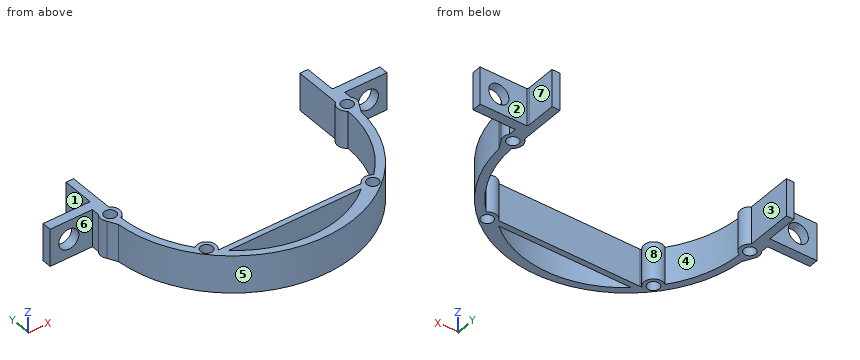
Autodesk Inventor part; units mm, degrees
ref_plane "YZ Plane" through (0, 0, 0) normal (1, 0, 0) x (0, 1, 0)
ref_plane "XZ Plane" through (0, 0, 0) normal (0, 1, 0) x (-1, 0, 0)
ref_plane "XY Plane" through (0, 0, 0) normal (0, 0, 1) x (1, 0, 0)
sketch "Esquisse1" plane through (0, 0, 0) normal (0, 0, 1) x (1, 0, 0)
  line L0 (0, 0) -> (-27.546, -25.0426) construction
  line L1 (0, 0) -> (23.0277, -27.4577) construction
  circle A0 centre (-18.0975, -16.4528) radius 1.25
  circle A1 centre (15.7127, -18.7355) radius 1.25
  arc A2 (-16.6894, -17.8731) -> (14.1299, -19.9581) centre (0, 0) ccw
  arc A3 (-16.6894, -17.8731) -> (-19.3824, -14.9201) centre (-18.0975, -16.4528) ccw
  arc A4 (17.0433, -17.2424) -> (14.1299, -19.9581) centre (15.7127, -18.7355) ccw
  line L2 (0, 0) -> (-29.5508, 10.7556) construction
  line L3 (-17.8311, 0) -> (17.1748, 0) construction
  line L4 (0, 2.0526) -> (0, -2.2236) construction
  arc A5 (-25.923, -2) -> (25.923, -2) centre (0, 0) ccw
  circle A6 centre (0, 0) radius 22.5 construction
  arc A7 (-16.6894, -17.8731) -> (14.1299, -19.9581) centre (0, 0) ccw
  arc A8 (-16.6894, -17.8731) -> (14.1299, -19.9581) centre (0, 0) ccw
  circle A9 centre (-25.3169, 1.1605) radius 1.25
  circle A10 centre (25.3169, 1.1605) radius 1.25
  line L5 (24.0891, 2.7784) -> (24.0891, 12.8348)
  line L6 (25.8363, 12.8348) -> (24.0891, 12.8348)
  line L7 (-25.923, 6.143) -> (-25.923, 12.7847)
  line L8 (-24.2942, 2.9148) -> (-24.2942, 12.7847)
  line L9 (-24.2942, 12.7847) -> (-25.923, 12.7847)
  arc A11 (-24.4506, -0.676) -> (-19.3824, -14.9201) centre (0, 0) ccw
  arc A12 (-24.4506, -0.676) -> (-19.3824, -14.9201) centre (0, 0) ccw
  arc A13 (-24.4506, -0.676) -> (-24.2942, 2.9148) centre (-25.3169, 1.1605) ccw
  arc A14 (17.0433, -17.2424) -> (24.2376, -0.5599) centre (0, 0) ccw
  arc A15 (17.0433, -17.2424) -> (24.2376, -0.5599) centre (0, 0) ccw
  arc A16 (17.0433, -17.2424) -> (24.2376, -0.5599) centre (0, 0) ccw
  arc A17 (24.0891, 2.7784) -> (24.2376, -0.5599) centre (25.3169, 1.1605) ccw
  line L10 (25.8363, 3.0919) -> (25.8363, 3.124)
  line L11 (25.8363, 6.3239) -> (25.8363, 12.8348)
  line L12 (25.8363, 6.3239) -> (25.9915, 6)
  line L13 (-36, 4) -> (-26.9495, 4)
  line L14 (-36, 6) -> (-26, 6)
  line L15 (-36, 4) -> (-36, 6)
  line L16 (-26, 6) -> (-25.9915, 6)
  line L17 (-25.9915, 6) -> (-25.923, 6.143)
  line L18 (-26.9495, 4) -> (-26.9495, 2.3678)
  line L19 (-25.923, -2) -> (-26.9495, -0.0468)
  arc A18 (-26.9495, 2.3678) -> (-26.9495, -0.0468) centre (-25.3169, 1.1605) ccw
  arc A19 (-24.4506, -0.676) -> (-24.2942, 2.9148) centre (-25.3169, 1.1605) ccw
  line L20 (25.9915, 6) -> (25.923, 6.143)
  line L21 (36, 4) -> (26.9495, 4)
  line L22 (36, 6) -> (26, 6)
  line L23 (36, 4) -> (36, 6)
  line L24 (26.9495, 4) -> (26.9495, 2.3678)
  line L25 (25.923, -2) -> (26.9495, -0.0468)
  arc A20 (26.9495, -0.0468) -> (26.9495, 2.3678) centre (25.3169, 1.1605) ccw
  line L26 (25.9915, 6) -> (26, 6)
  point P0 (29.8237, -2)
  point P1 (-36, -2)
  point P2 (-26.3114, 9.5766)
  dimension "d35" = 2.5
  dimension "d36" = 2.5
  dimension "d37" = 4
  dimension "d38" = 4
  dimension "d39" = 20
  dimension "d52" = 45
  dimension "d65" = 2.5
  dimension "d81" = 10
ref_plane "Plan de construction1" through (-42, 0, 0) normal (0, 1, 0) x (1, 0, 0)
ref_plane "Plan de construction2" through (-36, 0, 0) normal (0, 1, 0) x (1, 0, 0)
sketch "Esquisse3" plane through (-36, 0, 0) normal (0, 1, 0) x (1, 0, 0)
  line L0 (0, 0) -> (10, 0)
  line L1 (0, 0) -> (0, -8)
  line L2 (10, -8) -> (0, -8)
  line L3 (10, 0) -> (10, -8)
  circle A0 centre (4, -4) radius 2.15
  line L4 (62, 0) -> (72, 0)
  line L5 (62, 0) -> (62, -8)
  line L6 (72, -8) -> (62, -8)
  line L7 (72, 0) -> (72, -8)
  circle A1 centre (68, -4) radius 2.15
  point P0 (36, 0)
  dimension "d48" = 4.3
  dimension "d73" = 4
  dimension "d74" = 4.3
  dimension "d75" = 4
extrude "Extrusion16" add sketch "Esquisse1" along normal blind 8
extrude "Extrusion17" cut sketch "Esquisse3" along normal blind 8 contours A0 | A1
sketch "Esquisse5" plane through (0, 0, 8) normal (0, 0, 1) x (1, 0, 0)
  arc A0 (-16.6894, -17.8731) -> (14.1299, -19.9581) centre (0, 0) ccw
  circle A1 centre (25.3169, 1.1605) radius 1.25
  circle A2 centre (-25.3169, 1.1605) radius 1.25
  circle A3 centre (15.7127, -18.7355) radius 1.25
  circle A4 centre (-18.0975, -16.4528) radius 1.25
  arc A5 (-16.6894, -17.8731) -> (-19.3824, -14.9201) centre (-18.0975, -16.4528) ccw
  arc A6 (-24.4506, -0.676) -> (-19.3824, -14.9201) centre (0, 0) ccw
  arc A7 (-24.4506, -0.676) -> (-24.2942, 2.9148) centre (-25.3169, 1.1605) ccw
  line L0 (-24.2942, 2.9148) -> (-24.2942, 12.7847)
  line L1 (-24.2942, 12.7847) -> (-25.923, 12.7847)
  line L2 (-25.923, 12.7847) -> (-25.923, 6.143)
  line L3 (-25.923, 6.143) -> (-25.9915, 6)
  line L4 (-25.9915, 6) -> (-36, 6)
  line L5 (-36, 6) -> (-36, 4)
  line L6 (-36, 4) -> (-26.9495, 4)
  line L7 (-26.9495, 4) -> (-26.9495, 2.3678)
  arc A8 (-26.9495, 2.3678) -> (-26.9495, -0.0468) centre (-25.3169, 1.1605) ccw
  line L8 (-26.9495, -0.0468) -> (-25.923, -2)
  arc A9 (-25.923, -2) -> (25.923, -2) centre (0, 0) ccw
  line L9 (25.923, -2) -> (26.9495, -0.0468)
  arc A10 (26.9495, -0.0468) -> (26.9495, 2.3678) centre (25.3169, 1.1605) ccw
  line L10 (26.9495, 2.3678) -> (26.9495, 4)
  line L11 (26.9495, 4) -> (36, 4)
  line L12 (36, 4) -> (36, 6)
  line L13 (36, 6) -> (25.9915, 6)
  line L14 (25.9915, 6) -> (25.8363, 6.3239)
  line L15 (25.8363, 6.3239) -> (25.8363, 12.8348)
  line L16 (25.8363, 12.8348) -> (24.0891, 12.8348)
  line L17 (24.0891, 12.8348) -> (24.0891, 2.7784)
  arc A11 (24.0891, 2.7784) -> (24.2376, -0.5599) centre (25.3169, 1.1605) ccw
  arc A12 (17.0433, -17.2424) -> (24.2376, -0.5599) centre (0, 0) ccw
  arc A13 (17.0433, -17.2424) -> (14.1299, -19.9581) centre (15.7127, -18.7355) ccw
  arc A14 (-16.6894, -17.8731) -> (14.1299, -19.9581) centre (0, 0) ccw
  line L18 (-16.356, -17.8956) -> (-16.6894, -17.8731)
  arc A15 (17.0433, -17.2424) -> (14.1299, -19.9581) centre (15.7127, -18.7355) ccw
  arc A16 (13.8936, -17.9043) -> (-16.356, -17.8956) centre (-8.178, -24366.3326) ccw
  arc A17 (-16.6894, -17.8731) -> (-19.3824, -14.9201) centre (-18.0975, -16.4528) ccw
  arc A18 (-16.6894, -17.8731) -> (14.1299, -19.9581) centre (0, 0) ccw
  arc A19 (13.8936, -17.9043) -> (14.1299, -19.9581) centre (15.7127, -18.7355) ccw
extrude "Extrusion18" add sketch "Esquisse5" against normal blind 8 contours L18 A16 A13 A0
sketch "Esquisse6" plane through (0, 0, 8) normal (0, 0, 1) x (1, 0, 0)
  circle A0 centre (25.3169, 1.1605) radius 1.25
  circle A1 centre (-25.3169, 1.1605) radius 1.25
  circle A2 centre (15.7127, -18.7355) radius 1.25
  circle A3 centre (-18.0975, -16.4528) radius 1.25
  arc A4 (-16.6894, -17.8731) -> (-19.3824, -14.9201) centre (-18.0975, -16.4528) ccw
  arc A5 (-24.4506, -0.676) -> (-19.3824, -14.9201) centre (0, 0) ccw
  arc A6 (-24.4506, -0.676) -> (-24.2942, 2.9148) centre (-25.3169, 1.1605) ccw
  line L0 (-24.2942, 2.9148) -> (-24.2942, 12.7847)
  line L1 (-24.2942, 12.7847) -> (-25.923, 12.7847)
  line L2 (-25.923, 12.7847) -> (-25.923, 6.143)
  line L3 (-25.923, 6.143) -> (-25.9915, 6)
  line L4 (-25.9915, 6) -> (-36, 6)
  line L5 (-36, 6) -> (-36, 4)
  line L6 (-36, 4) -> (-26.9495, 4)
  line L7 (-26.9495, 4) -> (-26.9495, 2.3678)
  arc A7 (-26.9495, 2.3678) -> (-26.9495, -0.0468) centre (-25.3169, 1.1605) ccw
  line L8 (-26.9495, -0.0468) -> (-25.923, -2)
  arc A8 (-25.923, -2) -> (25.923, -2) centre (0, 0) ccw
  line L9 (25.923, -2) -> (26.9495, -0.0468)
  arc A9 (26.9495, -0.0468) -> (26.9495, 2.3678) centre (25.3169, 1.1605) ccw
  line L10 (26.9495, 2.3678) -> (26.9495, 4)
  line L11 (26.9495, 4) -> (36, 4)
  line L12 (36, 4) -> (36, 6)
  line L13 (36, 6) -> (25.9915, 6)
  line L14 (25.9915, 6) -> (25.8363, 6.3239)
  line L15 (25.8363, 6.3239) -> (25.8363, 12.8348)
  line L16 (25.8363, 12.8348) -> (24.0891, 12.8348)
  line L17 (24.0891, 12.8348) -> (24.0891, 2.7784)
  arc A10 (24.0891, 2.7784) -> (24.2376, -0.5599) centre (25.3169, 1.1605) ccw
  arc A11 (17.0433, -17.2424) -> (24.2376, -0.5599) centre (0, 0) ccw
  arc A12 (17.0433, -17.2424) -> (13.8936, -17.9043) centre (15.7127, -18.7355) ccw
  arc A13 (13.8936, -17.9043) -> (-16.356, -17.8956) centre (-8.178, -24366.3326) ccw
  line L18 (-16.356, -17.8956) -> (-16.6894, -17.8731)
  line L19 (-15.3155, -19.0715) -> (12.9977, -19.0715)
  arc A14 (-15.3155, -19.0715) -> (12.9977, -19.0715) centre (-1.1589, -2.415) ccw
extrude "Extrusion19" cut sketch "Esquisse6" against normal blind 8 contours L19 A14
properties part number "anneaustop"
Geometry check sheet. Reference: the model listing, model coordinates, mm. Face numbers are marked on the shaded views. A direction names the side the tool comes from. Round coordinates to 2 decimals unless told otherwise and drop trailing zeros. Write each loop counter-clockwise with the first axis right and the second up, starting at its lowest first coordinate (ties: lowest second). Pieces come first, ordered by that corner, then holes. Notation, with made-up numbers: (82.5, 24.25) - (124.5, 24.25) arc R4 ccw to (124.5, 29.25) - close; hole circle Ø1 at (-31, 7.5). An arc over 180 degrees is marked (long way). Write each question's results on one line, items separated by ' | '.
(1) Sectioned sample at C-C, the plane z = 4. Count the separate pieces of the cut face and the enclosed holes in it, plus the area to 3 significant figures.
Computed:
separate pieces: 3 | enclosed holes: 5 | area: 248 mm^2
(2) Sectioned sample at A-A, the plane x = -32. Enter the section's corners in (y, z).
Computed:
outline: (4, 0) - (6, 0) - (6, 1.85) - (4, 1.85) - close; (4, 6.15) - (6, 6.15) - (6, 8) - (4, 8) - close
(3) Sectioned sample at B-B, the plane y = 9. Enter the section's corners in (x, z), plus the area to 3 significant figures.
Computed:
outline: (-25.92, 0) - (-24.29, 0) - (-24.29, 8) - (-25.92, 8) - close; (24.09, 0) - (25.84, 0) - (25.84, 8) - (24.09, 8) - close | area: 27.0 mm^2
(4) Depth check by flat-ended pin: pin 1 Ø1 at (x, z) = (7.5, 7) entering from -Y; pin 2 Ø0.8 at (y, z) = (3, 4) entering from +X; pin 3 Ø1 at (y, z) = (-13, 1) entering from -X. Enter the tip coordinate at first touch or a pass-through.
Computed:
pin 1: stops at y = -25.04 | pin 2: stops at x = 26.95 | pin 3: stops at x = -22.8
(5) Set-up check for the marked faces 1, 2, 3 and 4: record each of +Z, -Z, +X, -X, +Y, -Y from which the full face is reachable in a straight line by a thin tool's end or side.
Computed:
face 1: +Z, -Z, -X, +Y | face 2: +Z, -Z, +X, +Y | face 3: +Z, -Z, +Y | face 4: +Z, -Z
(6) Thickness scan on probe 1 along Z at (x, y) = (32, 5); probe 2 along X at (y, z) = (-16, 3.25); probe 3 along X at (y, z) = (-6, 4). Record the ranges inside material, lowest first. Write a range as from..to.
Computed:
probe 1: z = 0..1.85, 6.15..8 | probe 2: x = -20.49..-19.26, -16.93..-16.15, 18.21..20.49 | probe 3: x = -25.3..-23.71, 23.49..25.3
(7) Draft check along X on the marked faces 5, 6, 7 and 8. Enter one of: pulls with the +X half, pulls with the -X half, needs draft (parallel to the pull), parting line crosses it, or undercut.
Computed:
face 5: parting line crosses it | face 6: needs draft | face 7: pulls with the +X half | face 8: undercut
